```python
from build123d import *

# Parameters (mm, degrees)
BOSS_EXTRUDE1_DEPTH = 6
BOSS_EXTRUDE2_DEPTH = 6
LPATTERN1_COUNT     = 15
LPATTERN1_PITCH     = 10


with BuildPart() as part:
    # Sketch1 → Boss-Extrude1 (new body)
    with BuildSketch(Plane.XY):
        Polygon((-75, 5), (-75, -5), (-72, -5), (-70, -5), (-67, -5), (-62, -5), (-60, -5), (-52, -5), (-50, -5), (-42, -5), (-40, -5), (-32, -5), (-30, -5), (-22, -5), (-20, -5), (-12, -5), (-10, -5), (-2, -5), (0, -5), (8, -5), (10, -5), (18, -5), (20, -5), (28, -5), (30, -5), (38, -5), (40, -5), (48, -5), (50, -5), (58, -5), (60, -5), (68, -5), (70, -5), (75, -5), (75, 5), align=None)
    extrude(amount=BOSS_EXTRUDE1_DEPTH)

    # Sketch2 → Boss-Extrude2 (add)
    with BuildSketch(Plane.XY.offset(6)):
        Polygon((-75, -5), (-72.125, -13), (-69.875, -13), (-67, -5), align=None)
    boss_extrude2 = extrude(amount=-BOSS_EXTRUDE2_DEPTH)

    # LPattern1: Boss-Extrude2 ×15
    with Locations(*[(i * LPATTERN1_PITCH, 0, 0) for i in range(1, LPATTERN1_COUNT)]):
        add(boss_extrude2)


solid = part.part
```
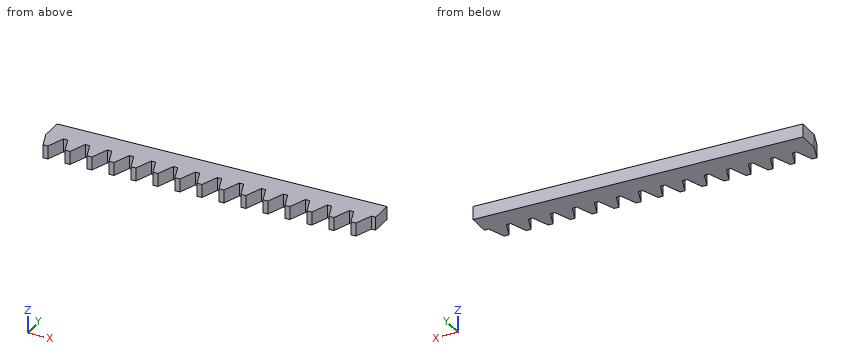
Geometry check sheet. Reference: the model listing, model coordinates, mm. Round coordinates to 2 decimals unless told otherwise and drop trailing zeros. Loops run counter-clockwise (first coordinate to the right, second up) from the corner with the lowest first, then second, coordinate; pieces in that order, holes last. Notation, with made-up numbers: M 38.25,40 L 57.25,40 A28 ccw 57.25,79 Z; hole C 26.25,-3.5 d1. An arc over 180 degrees is marked long. Return JSON: item names as keys, results as strings. Group by question number.
(1) Go/stop test with flat-tipped pins: pin 1 (1.6 mm diameter, centred on x = -66, z = 4, fed in from -Y); pin 2 (1.5 mm diameter, centred on y = -7, z = 4, fed in from +X). Record where each tip stops, or that it passes through.
(2) Section check A-A, the plane y = -6.25. Give the number of separate pieces and of enclosed holes in the cut face, and give its area (3 significant figures).
(3) Section check B-B, the plane x = -18.5. Enter the section's corners in (y, z).
Data:
{
 "1": {"pin 1": "y = -5", "pin 2": "x = 72.55"},
 "2": {"separate pieces": "15", "enclosed holes": "0", "area": "639 mm²"},
 "3": {"outline": "M -9.17,0 L 5,0 L 5,6 L -9.17,6 Z"}
}
